Verification items for this drawing (mm, ordinates from the low corner). A direction names the side the tool comes from. Coordinates: 2 decimals unless noted, no trailing zeros. Order: outer loops, then holes, each group sorted by start corner. A loop starts at its lowest first (then second) coordinate and runs counter-clockwise, first axis right, second up. Notation, with made-up numbers: M 85.5,79 L 112.5,79 A20 ccw 112.5,91 Z; hole C 37.25,-21 d9. An arc over 180 degrees is marked long. Write item = value, one per line.
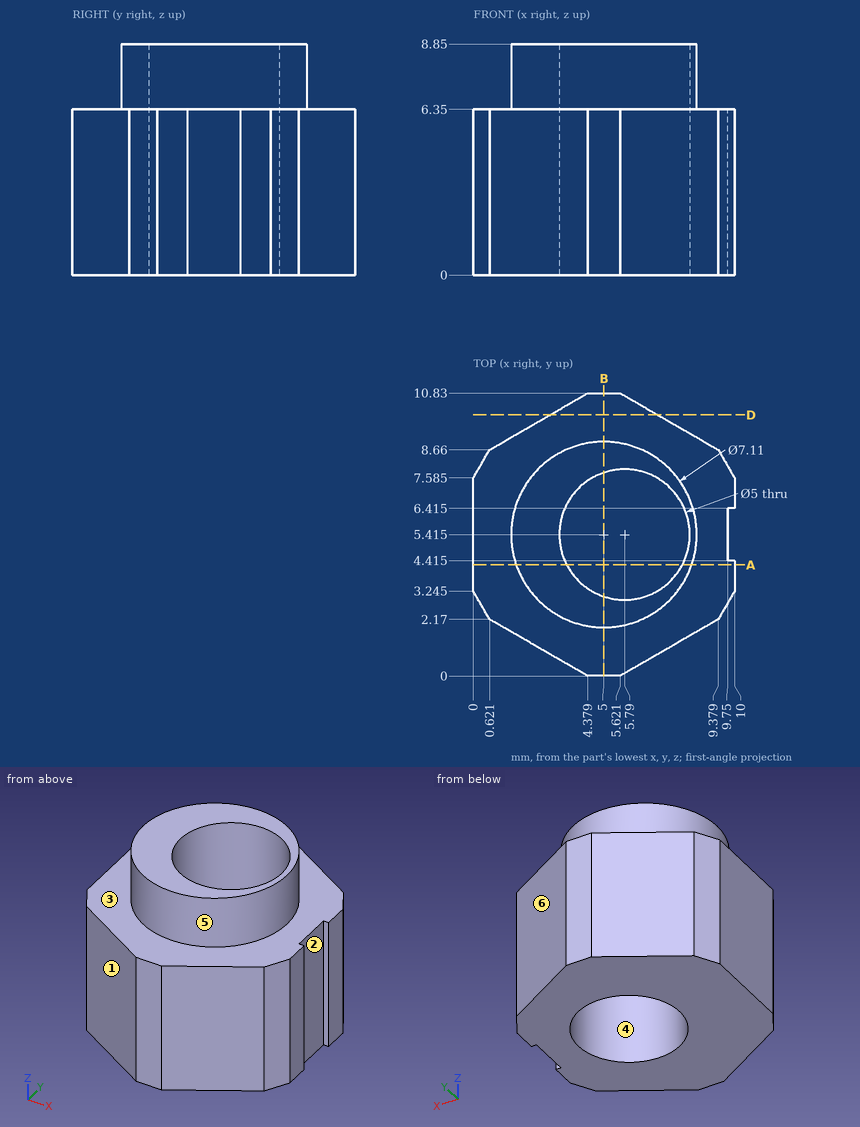
Item 1: Sectioned sample at D-D, the plane y = 10. Enter the section's corners in (x, z).
Report:
outline = M 2.94,0 L 7.06,0 L 7.06,6.35 L 2.94,6.35 Z
Item 2: Gauge pin test, flat ends, axial feed: pin 1 (2 mm diameter, centred on y = 7, z = 7.5, fed in from -X); pin 2 (1.5 mm diameter, centred on x = 1.5, z = 4, fed in from +Y); pin 3 (1 mm diameter, centred on x = 2.5, z = 7, fed in from -Y). Record the tip position at first contact, or that the pin passes through.
Report:
pin_1 = 1.49
pin_2 = 9.6
pin_3 = 2.48
Item 3: Sectioned sample at A-A, the plane y = 4.25. Enter the section's corners in (x, z).
Report:
outline = M 0,0 L 3.58,0 L 3.58,8.85 L 1.64,8.85 L 1.64,6.35 L 0,6.35 Z; M 8,0 L 10,0 L 10,6.35 L 8.36,6.35 L 8.36,8.85 L 8,8.85 Z
Item 4: Scan lines: L1, parallel to Y at x = 5.79, z = 2.75 (1 decimal); L2, parallel to Y at x = 7.5, z = 8.75; L3, parallel to X at y = 6.75, z = 8.25 (1 decimal). Record each from-to range of solid material in increasing order. Write a range as from..to.
Report:
L1 = 0.1..2.9, 7.9..10.7
L2 = 2.89..3.59, 7.24..7.94
L3 = 1.7..3.7, 7.9..8.3
Item 5: Tool access check on the marked faces 5 and 6. Record the directions out of +Z, -Z, +X, -X, +Y, -Y that give a thin tool (end or side, any length) a straight path to the whole face; none if there is none.
Report:
face_5 = +Z
face_6 = +Z, -Z, +X, +Y
Item 6: Sectioned sample at B-B, the plane x = 5. Enter the section's corners in (y, z).
Report:
outline = M 0,0 L 3.04,0 L 3.04,8.85 L 1.86,8.85 L 1.86,6.35 L 0,6.35 Z; M 7.79,0 L 10.83,0 L 10.83,6.35 L 8.97,6.35 L 8.97,8.85 L 7.79,8.85 Z
Item 7: Release check for a two-part mould opening along Y. For the marked faces 1, 2, 3 and 4 record: pulls with the +Y half, pulls with the -Y half, needs draft (parallel to the pull), parting line crosses it, or undercut.
Report:
face_1 = pulls with the -Y half
face_2 = undercut
face_3 = needs draft
face_4 = undercut
